Can you work these out from the model? Positions are in its coordinate system, mm. Give positions to 0.01 mm unless a question says otherwise; leave off trailing zeros. Loops run counter-clockwise (first coordinate to the right, second up) from the corner with the lowest first, then second, coordinate; pieces in that order, holes last. Notation, with made-up numbers: M 50.5,61 L 93.5,61 A22 cw 93.5,86 Z; hole C -12.5,43.5 d9. An arc over 180 degrees is marked long. Put each result on its own line as item: value. Start each with the question number.
1) Imagine slicing it at C-C (x = 18.5). Write out the boundary of the cut face in (y, z), then the cut area to 3 significant figures.
2) If we mould it in two halves opening along Z, with no side actions, what happens to faces 1 (the flat face through (-8, 3, -1)), 2 (the cylindrical face through (-22.818, 1.479, -29.759)), 3 (the cylindrical face through (-1.978, 1.479, -2.579)), 4 (the cylindrical face through (22.857, 1.479, 25.658))? For each: +Z half, -Z half, draft (parallel to the pull), parting line (faces both ways), or undercut.
3) For P1, Ø5, axis at x = 15, z = -0.5, coming from the -Y side; P2, Ø1.5, axis at x = -10.5, y = 0.5, coming from the -Z side, each with a flat end and sliding along its axis, tell me the tip position at first contact or that it passes through.
4) Imagine slicing it at B-B (y = 1.05). State how many separate pieces and enclosed holes the cut face has, then the cut area to 3 significant figures.
5) Please list where these lines run through material, in increasing order: line 1 along X through (y, z) = (2.3, 0); line 2 along X through (y, z) = (1.05, -6); line 3 along X through (y, z) = (0.2, -10.5). Write a range as from..to.
6) Imagine slicing it at A-A (z = 0). Write out the boundary of the cut face in (x, y).
7) Imagine slicing it at D-D (z = 31.5). Write out the boundary of the cut face in (x, y).
from build123d import *

# Parameters (mm, degrees)
SKETCH1_R           = 37.5
SKETCH1_R_2         = 0.75
SKETCH1_R_3         = 3.25
SKETCH1_R_4         = 1.5
BOSS_EXTRUDE1_DEPTH = 3


with BuildPart() as part:
    # Sketch1 → Boss-Extrude1 (new body)
    with BuildSketch(Plane(origin=(0, 0, 0), x_dir=(1, 0, 0), z_dir=(0, 1, 0))):
        with Locations(Location((0, 0, 0), (0, 0, 270))):
            Circle(SKETCH1_R)
        with Locations(Location((-0.863160321, 13.472377454, 0), (0, 0, 270))):
            Circle(SKETCH1_R_2, mode=Mode.SUBTRACT)
        with Locations(Location((-0.671346916, 10.478515797, 0), (0, 0, 270))):
            Circle(SKETCH1_R_2, mode=Mode.SUBTRACT)
        with Locations(Location((-0.479533512, 7.484654141, 0), (0, 0, 270))):
            Circle(SKETCH1_R_2, mode=Mode.SUBTRACT)
        with Locations(Location((6.242133869, 4.157615274, 0), (0, 0, 270))):
            Circle(SKETCH1_R_2, mode=Mode.SUBTRACT)
        with Locations(Location((8.738987416, 5.820661383, 0), (0, 0, 270))):
            Circle(SKETCH1_R_2, mode=Mode.SUBTRACT)
        with Locations(Location((11.235840964, 7.483707492, 0), (0, 0, 270))):
            Circle(SKETCH1_R_2, mode=Mode.SUBTRACT)
        with Locations(Location((-12.099001285, 5.988669961, 0), (0, 0, 270))):
            Circle(SKETCH1_R_2, mode=Mode.SUBTRACT)
        with Locations(Location((-9.410334333, 4.657854414, 0), (0, 0, 270))):
            Circle(SKETCH1_R_2, mode=Mode.SUBTRACT)
        with Locations(Location((-6.721667381, 3.327038867, 0), (0, 0, 270))):
            Circle(SKETCH1_R_2, mode=Mode.SUBTRACT)
        with Locations(Location((6.721667381, -3.327038867, 0), (0, 0, 270))):
            Circle(SKETCH1_R_2, mode=Mode.SUBTRACT)
        with Locations(Location((9.410334333, -4.657854414, 0), (0, 0, 270))):
            Circle(SKETCH1_R_2, mode=Mode.SUBTRACT)
        with Locations(Location((12.099001285, -5.988669961, 0), (0, 0, 270))):
            Circle(SKETCH1_R_2, mode=Mode.SUBTRACT)
        with Locations(Location((-11.235840964, -7.483707492, 0), (0, 0, 270))):
            Circle(SKETCH1_R_2, mode=Mode.SUBTRACT)
        with Locations(Location((-8.738987416, -5.820661383, 0), (0, 0, 270))):
            Circle(SKETCH1_R_2, mode=Mode.SUBTRACT)
        with Locations(Location((-6.242133869, -4.157615274, 0), (0, 0, 270))):
            Circle(SKETCH1_R_2, mode=Mode.SUBTRACT)
        with Locations(Location((0.479533512, -7.484654141, 0), (0, 0, 270))):
            Circle(SKETCH1_R_2, mode=Mode.SUBTRACT)
        with Locations(Location((0.671346916, -10.478515797, 0), (0, 0, 270))):
            Circle(SKETCH1_R_2, mode=Mode.SUBTRACT)
        with Locations(Location((0.863160321, -13.472377454, 0), (0, 0, 270))):
            Circle(SKETCH1_R_2, mode=Mode.SUBTRACT)
        with Locations(Location((0, 0, 0), (0, 0, 270))):
            Circle(SKETCH1_R_3, mode=Mode.SUBTRACT)
        with Locations(Location((-22.406587981, 24.226943989, 0), (0, 0, 270))):
            Circle(SKETCH1_R_4, mode=Mode.SUBTRACT)
        with Locations(Location((-30.815927231, 11.805872643, 0), (0, 0, 270))):
            Circle(SKETCH1_R_4, mode=Mode.SUBTRACT)
        with Locations(Location((30.815927231, -11.805872643, 0), (0, 0, 270))):
            Circle(SKETCH1_R_4, mode=Mode.SUBTRACT)
        with Locations(Location((22.406587981, -24.226943989, 0), (0, 0, 270))):
            Circle(SKETCH1_R_4, mode=Mode.SUBTRACT)
    extrude(amount=BOSS_EXTRUDE1_DEPTH)


solid = part.part
Recorded:
1. outline: M 0,-32.62 L 3,-32.62 L 3,32.62 L 0,32.62 Z
1. area: 196 mm²
2. face 1: draft
2. face 2: parting line
2. face 3: undercut
2. face 4: undercut
3. P1: y = 0
3. P2: z = -36.21
4. separate pieces: 1
4. enclosed holes: 23
4. area: 4,320 mm²
5. line 1: -37.5..-3.25, 3.25..37.5
5. line 2: -37.02..-12.85, -11.35..8.01, 9.47..37.02
5. line 3: -36..-31.55, -30.08..-1.42, 0.08..36
6. outline: M -37.5,0 L -3.25,0 L -3.25,3 L -37.5,3 Z; M 3.25,0 L 37.5,0 L 37.5,3 L 3.25,3 Z
7. outline: M -20.35,0 L 20.35,0 L 20.35,3 L -20.35,3 Z
